from build123d import *

# Parameters (mm, degrees)
F2_R     = 13.5
F2_R_2   = 11.5
F2_R_3   = 9
F2_R_4   = 7.5
F3_DEPTH = 2
F4_DEPTH = 25
F5_SIZE  = 1.49999
F6_SIZE  = 1


# Not quite as in the source:
# - a fillet or chamfer is up to 0.001 mm smaller than in the source, because OpenCascade refuses the exact size


with BuildPart() as f3:
    # F2 (on Top) → F3 (new body)
    with BuildSketch(Plane.XY):
        Circle(F2_R)
        Circle(F2_R_2, mode=Mode.SUBTRACT)
        Circle(F2_R_2)
        Circle(F2_R_3, mode=Mode.SUBTRACT)
        Circle(F2_R_3)
        Circle(F2_R_4, mode=Mode.SUBTRACT)
    extrude(amount=F3_DEPTH)

    # F2 (on Top) → F4 (join)
    with BuildSketch(Plane.XY):
        Circle(F2_R)
        Circle(F2_R_2, mode=Mode.SUBTRACT)
        Circle(F2_R_3)
        Circle(F2_R_4, mode=Mode.SUBTRACT)
    extrude(amount=F4_DEPTH)

    # F5 (size 1.5 in the source; OpenCascade refuses exactly that, so slightly less here)
    f5_edges = [f3.edges().sort_by_distance(p)[0] for p in [
        (-7.5, 0, 25),
    ]]
    chamfer(f5_edges, length=F5_SIZE)

    # F6
    f6_edges = [f3.edges().sort_by_distance(p)[0] for p in [
        (-13.5, 0, 25),
        (-13.5, 0, 0),
        (-7.5, 0, 0),
    ]]
    chamfer(f6_edges, length=F6_SIZE)


solid = f3.part
Read the model definition and answer for the solid it produces. Units are mm, in the model's axes. A direction names the side the tool comes from. Coordinates: 2 decimals unless noted, no trailing zeros. Order: outer loops, then holes, each group sorted by start corner. A loop starts at its lowest first (then second) coordinate and runs counter-clockwise, first axis right, second up. Notation, with made-up numbers: (39.25, 43.5) - (48.25, 43.5) arc R23 cw to (48.25, 67.5) - close; hole circle Ø3 at (49.5, 73.5). An arc over 180 degrees is marked (long way). Use one line per item in the form item = value.
(1) Given pin 1 Ø1.5 at (x, z) = (-5, 11) entering from +Y; pin 2 Ø12 at (y, z) = (8.5, 7.5) entering from -X; pin 3 Ø12 at (y, z) = (8, 4) entering from +X; pin 4 Ø5 at (y, z) = (2, 11) entering from -X, each flat-ended and moving along its own axis, determine where each tip first touches the part or whether it passes through.
Computed values:
pin_1 = 12.81
pin_2 = -13.27
pin_3 = 13.35
pin_4 = -13.5
(2) Straight lines are drawn through the part: L1, parallel to Y at x = 0, z = 16; L2, parallel to X at y = -5.75, z = 19.5; L3, parallel to X at y = -0.5, z = 21.25. For each, find the intervals that lie inside material, in ascending order.
Computed values:
L1 = -13.5 to -11.5, -9 to -7.5, 7.5 to 9, 11.5 to 13.5
L2 = -12.21 to -9.96, -6.92 to -4.82, 4.82 to 6.92, 9.96 to 12.21
L3 = -13.49 to -11.49, -8.99 to -7.48, 7.48 to 8.99, 11.49 to 13.49
(3) Section C-C, the plane z = 22.25 is taken. Give the vertices of the cut face in (x, y).
Computed values:
outline = circle Ø27 at (0, 0); circle Ø18 at (0, 0); hole circle Ø23 at (0, 0); hole circle Ø15 at (0, 0)
(4) For a pull along Y with two mould halves and no side action, classify faces 3 (the face through (-2.93, -13.18, 12.34)), 4 (the face through (-1.172, 8.923, 13.339)), 5 (the face through (-3, -8.2, 0)), 6 (the face through (-1.5, 11.4, 13.3)) as pulls with the +Y half, pulls with the -Y half, needs draft (parallel to the pull), parting line crosses it, or undercut.
Computed values:
face_3 = parting line crosses it
face_4 = undercut
face_5 = needs draft
face_6 = undercut
(5) Which of the six approach directions +Z, -Z, +X, -X, +Y, -Y give full straight-line access (tool end or side, diameter ignored) to faces 1 (the face through (-7, -6, 2)), 2 (the face through (-7.493, 0.33, 12.093))?
Computed values:
face_1 = +Z
face_2 = +Z, -Z
